CAD build for the part. Positions are in the model's coordinates, mm. Face numbers are marked on the shaded views. A direction names the side the tool comes from. Give positions to 0.01 mm unless a question says otherwise; leave off trailing zeros. Write each loop counter-clockwise with the first axis right and the second up, starting at its lowest first coordinate (ties: lowest second). Pieces come first, ordered by that corner, then holes. Notation, with made-up numbers: M -32,69.25 L 24,69.25 A17 ccw 24,99.25 Z; hole C -36,50.5 d4. An arc over 180 degrees is marked long. One line per question, with ' | ' between items. Start each with the question number.
1. Cut at D-D, the plane z = 2.5. Write the cut outline in (x, y), then the cut area to 3 significant figures.
2. Which spindle directions (+Z, -Z, +X, -X, +Y, -Y) get a long thin tool onto all of the face, cutting with end or side? Do the marked faces 1, 2 and 3. Say none if no direction does.
3. Flat gauge pins, fed straight in: pin 1 (8.5 mm diameter, centred on y = 15.5, z = 1, fed in from +X); pin 2 (1.5 mm diameter, centred on x = -14.5, z = 6, fed in from +Y); pin 3 (4 mm diameter, centred on y = 5.5, z = 0, fed in from +X); pin 4 (4.5 mm diameter, centred on y = 17, z = -3, fed in from -X). Where does each tip first touch, or does it go through?
4. Pull direction X, two halves, no side cores. Call the marked faces 4, 5, 6 and 7: released by +X, released by -X, zero draft, split by the parting line, or undercut.
5. Cut at A-A, the plane y = 17.5. Write the cut outline in (x, z), then the cut area to 3 significant figures.
6. Wall check: L1, parallel to Y at x = 5, z = 4.5; L2, parallel to Z at x = 0, y = 4.5; L3, parallel to X at y = 5.75, z = 0. Give the ranges that are in metal, low to high.
7. Cut at C-C, the plane y = 9.75. Write the cut outline in (x, z).
8. Cut at B-B, the plane x = 0. Write the cut outline in (y, z).
```python
from build123d import *

# Parameters (mm, degrees)
BASESKETCH_W       = 40
BASESKETCH_H       = 15
BASE_DEPTH         = 4
HOLDERSKETCH_W     = 18
HOLDERSKETCH_H     = 15
HOLDER_DEPTH       = 20
MOTORCUTSKETCH_W   = 14
MOTORCUTSKETCH_H   = 10.5
MOTORCUT_DEPTH     = 19
NUTTHOLE_DEPTH     = 4
HOLESKETCH_R       = 2
CUT_EXTRUDE3_DEPTH = 64


with BuildPart() as part:
    # BaseSketch → Base (new body)
    with BuildSketch(Plane(origin=(0, 0, 0), x_dir=(1, 0, 0), z_dir=(0, 1, 0))):
        Rectangle(BASESKETCH_W, BASESKETCH_H)
    extrude(amount=BASE_DEPTH)

    # HolderSketch → Holder (add)
    with BuildSketch(Plane(origin=(0, 4, 0), x_dir=(1, 0, 0), z_dir=(0, 1, 0))):
        Rectangle(HOLDERSKETCH_W, HOLDERSKETCH_H)
    extrude(amount=HOLDER_DEPTH)

    # MotorCutSketch → MotorCut (cut)
    with BuildSketch(Plane.XY.offset(7.5)):
        with Locations((0, 16.75)):
            Rectangle(MOTORCUTSKETCH_W, MOTORCUTSKETCH_H)
    extrude(amount=-MOTORCUT_DEPTH, mode=Mode.SUBTRACT)

    # NuttHoleSketch → NuttHole (cut)
    with BuildSketch(Plane(origin=(0, 11.5, 0), x_dir=(1, 0, 0), z_dir=(0, 1, 0))):
        Polygon((-2.309401077, 4), (-4.618802154, 0), (-2.309401077, -4), (2.309401077, -4), (4.618802154, 0), (2.309401077, 4), align=None)
    extrude(amount=-NUTTHOLE_DEPTH, mode=Mode.SUBTRACT)

    # HoleSketch → Cut-Extrude3 (cut)
    with BuildSketch(Plane(origin=(0, 7.5, 0), x_dir=(1, 0, 0), z_dir=(0, 1, 0))):
        Circle(HOLESKETCH_R)
    extrude(amount=-CUT_EXTRUDE3_DEPTH, mode=Mode.SUBTRACT)


solid = part.part
```
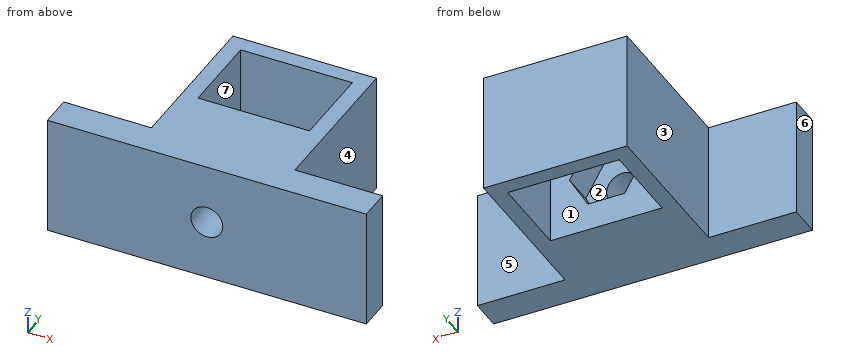
Here are the results:
1) outline: M -20,0 L 20,0 L 20,4 L 9,4 L 9,24 L -9,24 L -9,4 L -20,4 Z; hole M -7,11.5 L -3.18,11.5 L -3.18,7.5 L 3.18,7.5 L 3.18,11.5 L 7,11.5 L 7,22 L -7,22 Z | area: 348 mm^2
2) face 1: +Z, -Z | face 2: none | face 3: +Z, -Z, -X, +Y
3) pin 1: x = 9 | pin 2: y = 4 | pin 3: x = 20 | pin 4: x = -9
4) face 4: released by +X | face 5: zero draft | face 6: released by -X | face 7: undercut
5) outline: M -9,-7.5 L -7,-7.5 L -7,7.5 L -9,7.5 Z; M 7,-7.5 L 9,-7.5 L 9,7.5 L 7,7.5 Z | area: 60.0 mm^2
6) L1: 0 to 11.5, 22 to 24 | L2: -7.5 to -2, 2 to 7.5 | L3: -9 to -2, 2 to 9
7) outline: M -9,-7.5 L 9,-7.5 L 9,7.5 L -9,7.5 Z; hole M -4.62,0 L -2.31,-4 L 2.31,-4 L 4.62,0 L 2.31,4 L -2.31,4 Z
8) outline: M 0,-7.5 L 11.5,-7.5 L 11.5,-4 L 7.5,-4 L 7.5,-2 L 0,-2 Z; M 0,2 L 7.5,2 L 7.5,4 L 11.5,4 L 11.5,7.5 L 0,7.5 Z; M 22,-7.5 L 24,-7.5 L 24,7.5 L 22,7.5 Z
